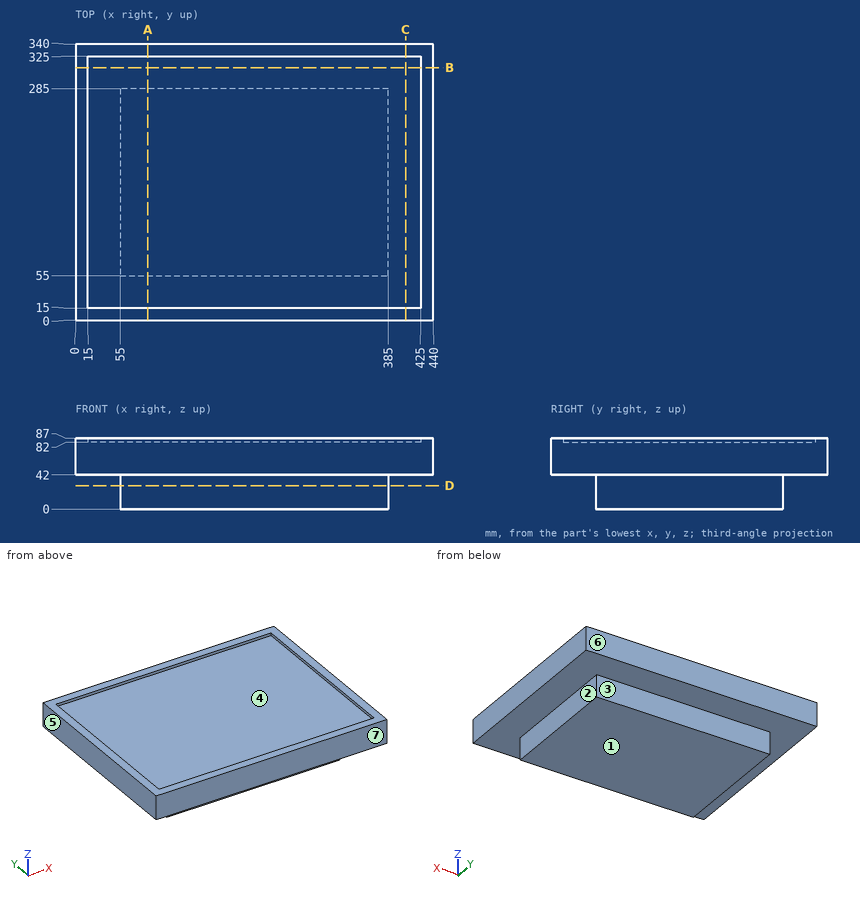
Geometry check sheet. Reference: drawing and pictorial views, mm from the part's lowest x, y, z. A direction names the side the tool comes from. Coordinates: 2 decimals unless noted, no trailing zeros. Write each loop counter-clockwise with the first axis right and the second up, starting at its lowest first coordinate (ties: lowest second). Pieces come first, ordered by that corner, then holes. Notation, with made-up numbers: M 71,45 L 81,45 A23 cw 81,72 Z; hole C -14,7.25 d9. An arc over 180 degrees is marked long. One line per question, with ' | ' between items.
1) Access from +Z, -Z, +X, -X, +Y, -Y to the whole of each face (thin tool, end or side, straight path). Record for the marked faces 1, 2 and 3.
Solutions:
face 1: -Z, +X, -X, +Y, -Y | face 2: -Z, +X, +Y, -Y | face 3: -Z, +X, -X, +Y
2) Sectioned sample at D-D on z = 29. Record the cut outline in (x, y).
Solutions:
outline: M 55,55 L 385,55 L 385,285 L 55,285 Z
3) Depth check by flat-ended pin: pin 1 Ø6 at (x, y) = (346, 199) entering from +Z; pin 2 Ø8 at (x, z) = (194, 15) entering from +Y; pin 3 Ø21 at (x, z) = (276, 12.5) entering from -Y. Enter the tip coordinate at first touch or a pass-through.
Solutions:
pin 1: z = 82 | pin 2: y = 285 | pin 3: y = 55
4) Sectioned sample at C-C on x = 406. Record the cut outline in (y, z), then the cut area to 4 significant figures.
Solutions:
outline: M 0,42 L 340,42 L 340,87 L 325,87 L 325,82 L 15,82 L 15,87 L 0,87 Z | area: 13,750 mm^2
5) Release check for a two-part mould opening along Y. For the marked faces 4, 5, 6 and 7 record: +Y half, -Y half, draft (parallel to the pull), parting line (faces both ways), or undercut.
Solutions:
face 4: undercut | face 5: draft | face 6: +Y half | face 7: -Y half
6) Material ranges on L1, parallel to Z at x = 206, y = 175.5; L2, parallel to Y at x = 231, z = 12; L3, parallel to Z at x = 62.5, y = 48, recorded low to high.
Solutions:
L1: 0 to 82 | L2: 55 to 285 | L3: 42 to 82
7) Sectioned sample at A-A on x = 89. Record the cut outline in (y, z), then the cut area to 3 significant figures.
Solutions:
outline: M 0,42 L 55,42 L 55,0 L 285,0 L 285,42 L 340,42 L 340,87 L 325,87 L 325,82 L 15,82 L 15,87 L 0,87 Z | area: 23,400 mm^2
8) Sectioned sample at B-B on y = 311. Record the cut outline in (x, z).
Solutions:
outline: M 0,42 L 440,42 L 440,87 L 425,87 L 425,82 L 15,82 L 15,87 L 0,87 Z
